Build history of the part. All positions in model axes, mm. Coordinates: 2 decimals unless noted, no trailing zeros. Write each loop counter-clockwise with the first axis right and the second up, starting at its lowest first coordinate (ties: lowest second). Pieces come first, ordered by that corner, then holes.
```python
from build123d import *

# Parameters (mm, degrees)
IZIM2_R                     = 15.5
IZIM2_R_2                   = 2.05
Y_KSEKLIK_EKSTR_ZYON1_DEPTH = 1
IZIM3_W                     = 1.5
IZIM3_H                     = 0.75
IZIM3_R                     = 0.25
IZIM3_W_2                   = 0.75
IZIM3_H_2                   = 1.5
Y_KSEKLIK_EKSTR_ZYON2_DEPTH = 0.25
KES_EKSTR_ZYON1_DEPTH       = 22.943108257
KES_EKSTR_ZYON1_DEPTH_BACK  = 22.943108257
IZIM3_3_R                   = 0.25


with BuildPart() as part:
    # Çizim2 → Yükseklik-Ekstrüzyon1 (new body)
    with BuildSketch(Plane.XY.offset(2)):
        Circle(IZIM2_R)
        Circle(IZIM2_R_2, mode=Mode.SUBTRACT)
    extrude(amount=Y_KSEKLIK_EKSTR_ZYON1_DEPTH)

    # Çizim3 → Yükseklik-Ekstrüzyon2 (add)
    # profile 1 of 2: a face of its own
    with BuildSketch(Plane.XY.offset(3)):
        with Locations((2.765409388, 0)):
            Rectangle(IZIM3_W, IZIM3_H)
        with Locations((2.765409388, 0)):
            Circle(IZIM3_R, mode=Mode.SUBTRACT)
    # profile 2 of 2: a face of its own
    with BuildSketch(Plane.XY.offset(3)):
        with Locations((0, -2.765409388)):
            Rectangle(IZIM3_W_2, IZIM3_H_2)
        with Locations((0, -2.765409388)):
            Circle(IZIM3_R, mode=Mode.SUBTRACT)
    extrude(amount=Y_KSEKLIK_EKSTR_ZYON2_DEPTH)

    # Çizim3<3> → Kes-Ekstrüzyon1 (cut, two sides: drawn at the far end of the back side and taken through both)
    with BuildSketch(Plane.XY.offset(3).offset(-KES_EKSTR_ZYON1_DEPTH_BACK)):
        with Locations((0, -2.765409388)):
            Circle(IZIM3_3_R)
        with Locations((2.765409388, 0)):
            Circle(IZIM3_3_R)
    extrude(amount=KES_EKSTR_ZYON1_DEPTH + KES_EKSTR_ZYON1_DEPTH_BACK, mode=Mode.SUBTRACT)


solid = part.part
```
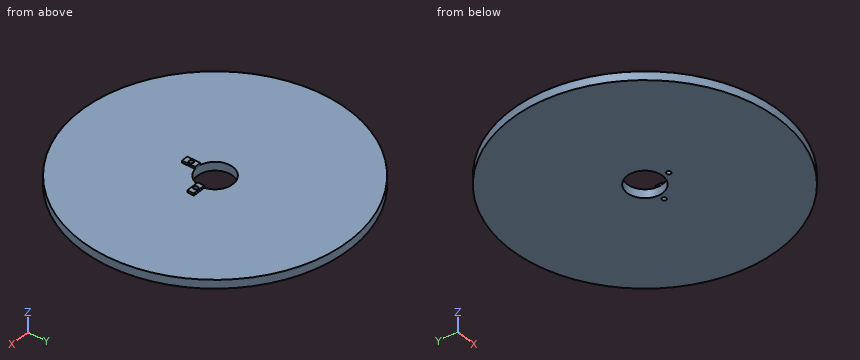
1. Saw through at B-B on y = 3. List the corners of the cut face in (x, z).
Computed values:
outline: (-15.21, 2) - (15.21, 2) - (15.21, 3) - (-15.21, 3) - close
2. Saw through at D-D on x = -7. List the corners of the cut face in (y, z), plus the area to 3 significant figures.
Computed values:
outline: (-13.83, 2) - (13.83, 2) - (13.83, 3) - (-13.83, 3) - close
area: 27.7 mm2
3. Saw through at A-A on x = -1. List the corners of the cut face in (y, z).
Computed values:
outline: (-15.47, 2) - (-1.79, 2) - (-1.79, 3) - (-15.47, 3) - close; (1.79, 2) - (15.47, 2) - (15.47, 3) - (1.79, 3) - close
4. Probe line 1 along Y through (x, z) = (0, 2.6); line 2 along Z through (x, y) = (1.5, -9.5); line 3 along X through (y, z) = (0.5, 2.1). List the from-to ranges inside material, lowest first.
Computed values:
line 1: y = -15.5 to -3.02, -2.52 to -2.05, 2.05 to 15.5
line 2: z = 2 to 3
line 3: x = -15.49 to -1.99, 1.99 to 15.49
5. Saw through at C-C on z = 2.6. List the corners of the cut face in (x, y), plus the area to 3 significant figures.
Computed values:
outline: circle Ø31 at (0, 0); hole circle Ø4.1 at (0, 0); hole circle Ø0.5 at (0, -2.77); hole circle Ø0.5 at (2.77, 0)
area: 741 mm2
